Source: CAD feature listing. Evaluate the final solid. Frame: model axes, mm. A direction names the side the tool comes from. Round coordinates to 2 decimals unless told otherwise and drop trailing zeros. Answer in a Markdown table with one row per item. Add a question column.
Item 1: Set-up query: faces 1 (the face through (-5, -50.8, 5)), 2 (the face through (-11.75, -73.34, 46.82)), 3 (the face through (-46, -50.8, 45)). Return all of +Z, -Z, +X, -X, +Y, -Y with unobstructed straight access to the full face (end or side cutting, diameter ignored); none if empty.
Item 2: Material intervals for probe 1 along Y at (x, z) = (-10.5, 46); probe 2 along Z at (x, y) = (-13.5, -54.5); probe 3 along Z at (x, y) = (-5.5, -82), sorted ascending.
Item 3: Contact query for a flat-ended pin moving along its axis: pin 1 (8 mm diameter, centred on x = -5.5, y = -56.5, fed in from -Z). Output: stop coordinate, or through.
from build123d import *

# Parameters (mm, degrees)
F0_W     = 50.8
F0_H     = 50.8
F1_DEPTH = 50.8
F2_R     = 25.4
F3_DEPTH = 50.8
F4_R     = 5.08
F5_R     = 5.08


with BuildPart() as f1:
    # F0 (on Front) → F1 (new body)
    with BuildSketch(Plane.XZ):
        with Locations((-25.4, 25.4)):
            Rectangle(F0_W, F0_H)
    extrude(amount=F1_DEPTH)

    # F2 (on face) → F3 (join)
    with BuildSketch(Plane.XZ.offset(50.8)):
        with Locations((-25.4, 25.4)):
            Circle(F2_R)
    extrude(amount=F3_DEPTH)

    # F4
    f4_edges = [f1.edges().sort_by_distance(p)[0] for p in [
        (-25.4, 0, 0),
        (0, 0, 25.4),
        (-25.4, 0, 50.8),
        (-50.8, 0, 25.4),
    ]]
    fillet(f4_edges, radius=F4_R)

    # F5
    f5_edges = [f1.edges().sort_by_distance(p)[0] for p in [
        (-50.8, -101.6, 25.4),
    ]]
    fillet(f5_edges, radius=F5_R)


solid = f1.part
Results below:
| question | item | result |
|---|---|---|
| 1 | face 1 | -Z, +X, -Y |
| 1 | face 2 | -Y |
| 1 | face 3 | +Z, -X, -Y |
| 2 | probe 1 | -50.8 to -0.01 |
| 2 | probe 2 | 2.96 to 47.84 |
| 2 | probe 3 | 9.62 to 41.18 |
| 3 | pin 1 | z = 5.59 |
